The listing builds one solid part. Answer for the finished solid, in the listing's coordinates (mm). A direction names the side the tool comes from. Coordinates: 2 decimals unless noted, no trailing zeros. Order: outer loops, then holes, each group sorted by start corner. A loop starts at its lowest first (then second) coordinate and runs counter-clockwise, first axis right, second up.
Autodesk Inventor part; units mm, degrees
ref_plane "YZ Plane" through (0, 0, 0) normal (1, 0, 0) x (0, 1, 0)
ref_plane "XZ Plane" through (0, 0, 0) normal (0, 1, 0) x (-1, 0, 0)
ref_plane "XY Plane" through (0, 0, 0) normal (0, 0, 1) x (1, 0, 0)
sketch "Sketch1" plane through (0, 0, 0) normal (0, 1, 0) x (-1, 0, 0)
  circle A0 centre (0, 0) radius 13.5
  circle A1 centre (0, 0) radius 16.5
  dimension "d0" = 27
  dimension "d1" = 33
extrude "pipeEnd" add sketch "Sketch1" along normal blind 17
sketch "Sketch2" plane through (0, 0, 0) normal (0, 1, 0) x (-1, 0, 0)
  circle A0 centre (0, 0) radius 19.5 construction
  line L0 (16.8875, -9.75) -> (16.8875, 9.75)
  line L1 (16.8875, 9.75) -> (0, 19.5)
  line L2 (0, 19.5) -> (-16.8875, 9.75)
  line L3 (-16.8875, 9.75) -> (-16.8875, -9.75)
  line L4 (-16.8875, -9.75) -> (0, -19.5)
  line L5 (0, -19.5) -> (16.8875, -9.75)
  circle A1 centre (0, 0) radius 11
  dimension "d4" = 39
  dimension "d12" = 22
extrude "hexBit" add sketch "Sketch2" against normal blind 6
sketch "Sketch3" plane through (0, -6, 0) normal (0, -1, 0) x (1, 0, 0)
  circle A0 centre (0, 0) radius 9
  circle A1 centre (0, 0) radius 13
  dimension "d7" = 18
  dimension "d8" = 26
extrude "thread" add sketch "Sketch3" along normal blind 15
thread "Thread1"
sketch "pinsPlacement" plane through (0, -21, 0) normal (0, -1, 0) x (1, 0, 0)
  point P0 (0, 0)
  point P1 (0, 0)
properties part number "PVCConnectorMale3_4inch"
(1) Find section A-A on z = 0. Determine the outline of the cut face in (x, y), then the cut area to 3 significant figures.
(2) Find the intervals of material crossed by probe 1 along Z at (x, y) = (0, 13.5); probe 2 along Z at (x, y) = (0, -11.25); probe 3 along Y at (x, z) = (-11, -2.5), in increasing order.
(3) Find section D-D on x = -10. Determine the outline of the cut face in (y, z), then the cut area to 3 significant figures.
(4) A tool of negligible diameter and unlimited length cuts with its end or side. For faces 1 (the flat face through (1.3, -6, 13.1)), 2 (the flat face through (5, 0, -10)), 3 (the flat face through (8.56, -2.96, -14.56)), from which of +Z, -Z, +X, -X, +Y, -Y can it reach the whole face along a straight path? Write none if from no direction.
(5) Given pin 1 Ø10 at (x, y) = (-11.5, -7) entering from -Z; pin 2 Ø3 at (y, z) = (2.5, -8.5) entering from -X; pin 3 Ø3 at (x, y) = (-4.5, 12) entering from +Z (3 decimals), each flat-ended and moving along its own axis, determine where each tip first touches the part or whether it passes through.
(6) Find section C-C on y = 6. Determine the outline of the cut face in (x, z).
(7) Find section B-B on x = -2. Determine the outline of the cut face in (y, z).
Resolved:
1. outline: (-16.89, -6) - (-13, -6) - (-13, -21) - (-9, -21) - (-9, -6) - (-11, -6) - (-11, 0) - (-13.5, 0) - (-13.5, 17) - (-16.5, 17) - (-16.5, 0) - (-16.89, 0) - close; (9, -21) - (13, -21) - (13, -6) - (16.89, -6) - (16.89, 0) - (16.5, 0) - (16.5, 17) - (13.5, 17) - (13.5, 0) - (11, 0) - (11, -6) - (9, -6) - close
1. area: 293 mm2
2. probe 1: z = -16.5 to -13.5, 13.5 to 16.5
2. probe 2: z = -13 to -9, 9 to 13
2. probe 3: y = -21 to 0
3. outline: (-21, -8.31) - (-6, -8.31) - (-6, -13.73) - (0, -13.73) - (0, -13.12) - (17, -13.12) - (17, -9.07) - (0, -9.07) - (0, -4.58) - (-6, -4.58) - (-6, 4.58) - (0, 4.58) - (0, 9.07) - (17, 9.07) - (17, 13.12) - (0, 13.12) - (0, 13.73) - (-6, 13.73) - (-6, 8.31) - (-21, 8.31) - close
3. area: 497 mm2
4. face 1: -Y
4. face 2: +Y
4. face 3: -Z, +X, +Y, -Y
5. pin 1: stops at z = -15.69
5. pin 2: stops at x = -14.94
5. pin 3: stops at z = 16.225
6. outline: circle Ø33 at (0, 0); hole circle Ø27 at (0, 0)
7. outline: (-21, -12.85) - (-6, -12.85) - (-6, -18.35) - (0, -18.35) - (0, -16.38) - (17, -16.38) - (17, -13.35) - (0, -13.35) - (0, -10.82) - (-6, -10.82) - (-6, -8.77) - (-21, -8.77) - close; (-21, 8.77) - (-6, 8.77) - (-6, 10.82) - (0, 10.82) - (0, 13.35) - (17, 13.35) - (17, 16.38) - (0, 16.38) - (0, 18.35) - (-6, 18.35) - (-6, 12.85) - (-21, 12.85) - close
